Can you work these out from the drawing? Everything is in mm from the part's minimum corner. Give positions to 0.01 mm unless a question says otherwise; leave off trailing zeros. Write each loop counter-clockwise with the first axis right and the second up, starting at its lowest first coordinate (ties: lowest second). Pieces come first, ordered by that corner, then holes. Notation, with made-up numbers: M 66,61.5 L 124,61.5 A25 ccw 124,87.5 Z; hole C 74.5,28.25 d9. An arc over 180 degrees is marked long. One line per item, written item: value.
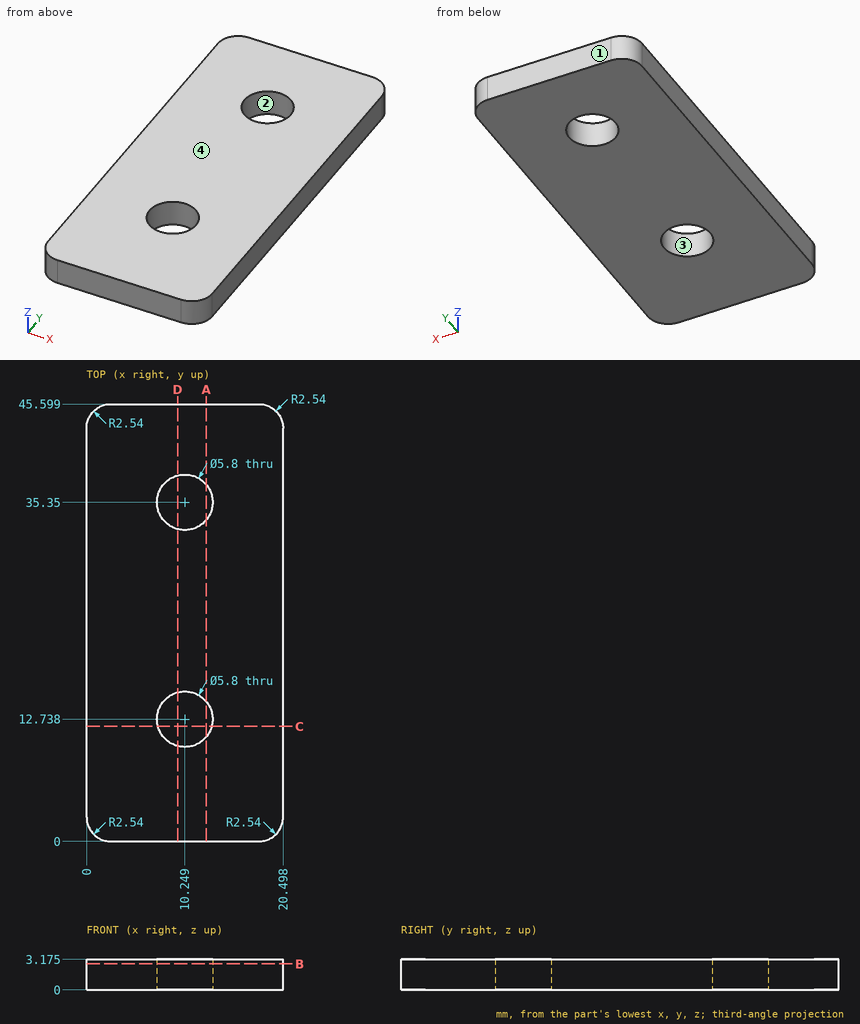
1) I'm going to push a flat-ended pin straight in: pin 1 (7.5 mm diameter, centred on x = 10.25, y = 35.35, fed in from +Z) (3 decimals). Where does the tip first touch, or does it pass through?
Outcome:
pin 1: stops at z = 3.175
2) If we section it at C-C, the plane y = 12: Write out the boundary of the cut face in (x, z) (1 decimal).
Outcome:
outline: M 0,0 L 7.4,0 L 7.4,3.2 L 0,3.2 Z; M 13.1,0 L 20.5,0 L 20.5,3.2 L 13.1,3.2 Z
3) Please list where these lines run through material, in increasing order: L1, parallel to Y at x = 11, z = 2.4; L2, parallel to Y at x = 9, z = 2.1 (1 decimal); L3, parallel to X at y = 12, z = 2.25 (1 decimal). Write a range as from..to.
Outcome:
L1: y = 0..9.94, 15.54..32.55, 38.15..45.6
L2: y = 0..10.1, 15.4..32.7, 38..45.6
L3: x = 0..7.4, 13.1..20.5
4) We'd pull the mould along Y, two halves only. Please class the marked faces 1, 2, 3 and 4: pulls with the +Y half, pulls with the -Y half, needs draft (parallel to the pull), parting line crosses it, or undercut.
Outcome:
face 1: pulls with the +Y half
face 2: undercut
face 3: undercut
face 4: needs draft
5) If we section it at B-B, the plane z = 2.7: Write out the boundary of the cut face in (x, y).
Outcome:
outline: M 0,2.54 A2.54 ccw 2.54,0 L 17.96,0 A2.54 ccw 20.5,2.54 L 20.5,43.06 A2.54 ccw 17.96,45.6 L 2.54,45.6 A2.54 ccw 0,43.06 Z; hole C 10.25,12.74 d5.8; hole C 10.25,35.35 d5.8
6) If we section it at A-A, the plane x = 12.5: Write out the boundary of the cut face in (y, z) (1 decimal).
Outcome:
outline: M 0,0 L 10.9,0 L 10.9,3.2 L 0,3.2 Z; M 14.6,0 L 33.5,0 L 33.5,3.2 L 14.6,3.2 Z; M 37.2,0 L 45.6,0 L 45.6,3.2 L 37.2,3.2 Z
7) If we section it at D-D, the plane x = 9.5: Write out the boundary of the cut face in (y, z) (1 decimal), then the cut area to 3 significant figures.
Outcome:
outline: M 0,0 L 9.9,0 L 9.9,3.2 L 0,3.2 Z; M 15.5,0 L 32.5,0 L 32.5,3.2 L 15.5,3.2 Z; M 38.2,0 L 45.6,0 L 45.6,3.2 L 38.2,3.2 Z
area: 109 mm^2
